Part model, mm, in its own coordinate system. Face numbers are marked on the shaded views. Round coordinates to 2 decimals unless told otherwise and drop trailing zeros. Order: outer loops, then holes, each group sorted by start corner. A loop starts at its lowest first (then second) coordinate and runs counter-clockwise, first axis right, second up. Notation, with made-up numbers: (-16.75, 23.5) - (32.25, 23.5) arc R29 ccw to (32.25, 52.5) - close; hole circle Ø8 at (-15, 63). An arc over 180 degrees is marked (long way). Answer as a JSON object with one key per item and string values.
```python
from build123d import *

# Parameters (mm, degrees)
ESQUISSE2_R                                    = 76.2
ESQUISSE2_R_2                                  = 50.8
BOSS_EXTRU_1_DEPTH                             = 10
CHANFREIN1_SIZE                                = 2
D_GAGEMENT_81_D                                = 4.4958
FRAISAGE_POUR_VIS_T_TE_FRAIS_E_M51_D           = 5.5
FRAISAGE_POUR_VIS_T_TE_FRAIS_E_M51_CSINK_D     = 10.4
FRAISAGE_POUR_VIS_T_TE_FRAIS_E_M51_CSINK_ANGLE = 90


with BuildPart() as part:
    # Esquisse2 → Boss.-Extru.1 (new body)
    with BuildSketch(Plane.XY):
        Circle(ESQUISSE2_R)
        Circle(ESQUISSE2_R_2, mode=Mode.SUBTRACT)
    extrude(amount=BOSS_EXTRU_1_DEPTH)

    # Chanfrein1
    chanfrein1_edges = [part.edges().sort_by_distance(p)[0] for p in [
        (-76.2, 0, 0),
    ]]
    chamfer(chanfrein1_edges, length=CHANFREIN1_SIZE)

    # Dégagement #81 (through all)
    with Locations(Plane(origin=(0, 0, 0), x_dir=(-1, 0, 0), z_dir=(0, 0, -1))):
        with Locations((0, 59.65), (51.658415336, 29.825), (29.825, 51.658415336), (59.65, 0), (51.658415336, -29.825), (29.825, -51.658415336), (0, -59.65), (-29.825, -51.658415336), (-51.658415336, -29.825), (-59.65, 0), (-51.658415336, 29.825), (-29.825, 51.658415336)):
            Hole(D_GAGEMENT_81_D / 2)

    # Fraisage pour vis à tête fraisée M51 (through all)
    with Locations(Plane(origin=(0, 0, 0), x_dir=(-1, 0, 0), z_dir=(0, 0, -1))):
        with Locations((68.1, 0), (-35.565, -59.851015656), (-35.565, 59.851015656)):
            CounterSinkHole(FRAISAGE_POUR_VIS_T_TE_FRAIS_E_M51_D / 2, FRAISAGE_POUR_VIS_T_TE_FRAIS_E_M51_CSINK_D / 2, counter_sink_angle=FRAISAGE_POUR_VIS_T_TE_FRAIS_E_M51_CSINK_ANGLE)


solid = part.part
```
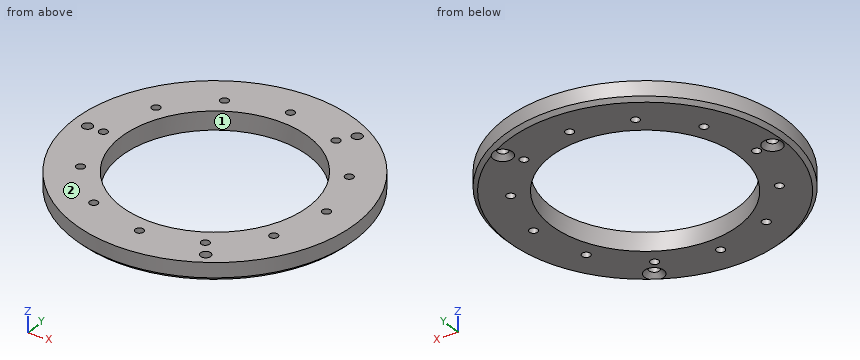
Item 1: Drop flat-ended pins along their axis: P1, Ø6, axis at x = 19.5, z = 7, coming from the +Y side; P2, Ø2, axis at x = -40, z = 8, coming from the -Y side; P3, Ø3, axis at y = -2, z = 6, coming from the -X side. Give the stop position or say it passes through.
Taken from the geometry:
{"P1": "y = 74.39", "P2": "y = -65.46", "P3": "x = -76.2"}
Item 2: Cut at A-A (y = 0). Write the cut outline in (x, z), plus the area to 3 significant figures.
Taken from the geometry:
{"outline": "(-76.2, 2) - (-74.2, 0) - (-73.3, 0) - (-70.85, 2.45) - (-70.85, 10) - (-76.2, 10) - close; (-65.35, 2.45) - (-62.9, 0) - (-61.9, 0) - (-61.9, 10) - (-65.35, 10) - close; (-57.4, 0) - (-50.8, 0) - (-50.8, 10) - (-57.4, 10) - close; (50.8, 0) - (57.4, 0) - (57.4, 10) - (50.8, 10) - close; (61.9, 0) - (74.2, 0) - (76.2, 2) - (76.2, 10) - (61.9, 10) - close", "area": "353 mm2"}
Item 3: Two-plate mould, pull along Y, no slides. Class the marked faces 1 and 2: pulls with the +Y half, pulls with the -Y half, needs draft (parallel to the pull), parting line crosses it, or undercut.
Taken from the geometry:
{"face 1": "undercut", "face 2": "needs draft"}
Item 4: Cut at B-B (z = 7.25). State how many separate pieces and enclosed holes the cut face has, plus the area to 3 significant figures.
Taken from the geometry:
{"separate pieces": "1", "enclosed holes": "16", "area": "9,870 mm2"}
Item 5: Probe L1, parallel to Y at x = 0, z = 6.25; L2, parallel to X at y = -23, z = 2; L3, parallel to X at y = 37.5, z = 5. List the from-to ranges inside material, lowest first. Write a range as from..to.
Taken from the geometry:
{"L1": "-76.2..-61.9, -57.4..-50.8, 50.8..57.4, 61.9..76.2", "L2": "-72.65..-45.3, 45.3..72.65", "L3": "-66.33..-34.27, 34.27..66.33"}
